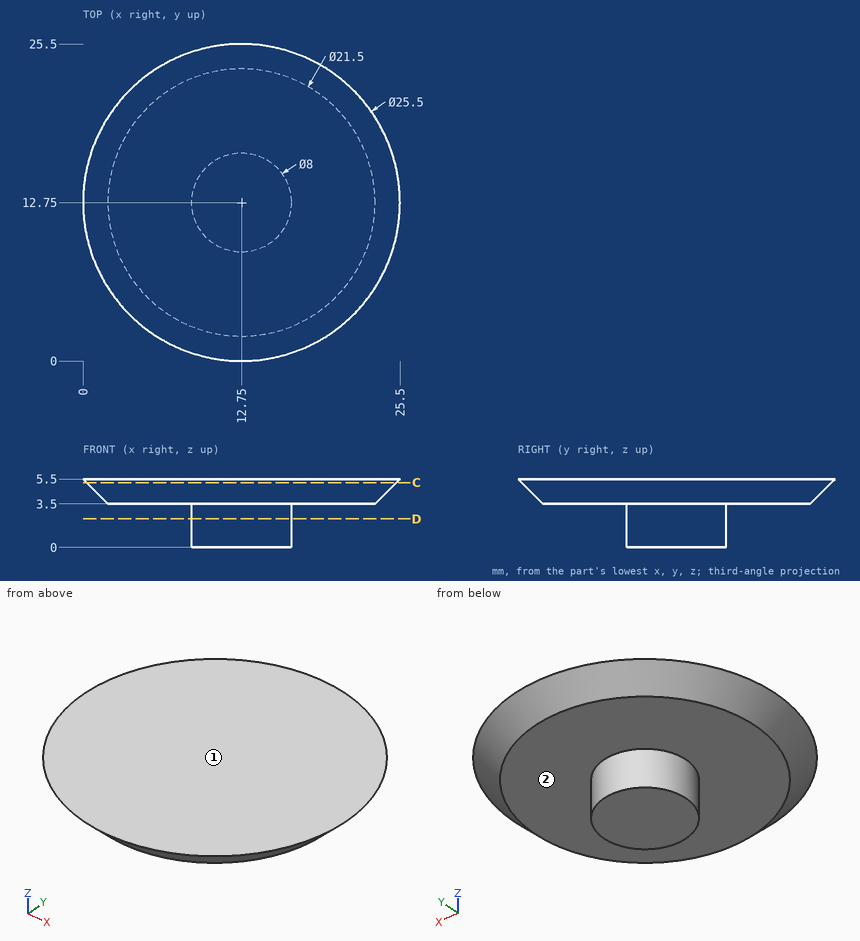
Input: dimensioned drawing with shaded views. Units: mm. Origin: part minimum x, y, z. A direction names the side the tool comes from. Give positions to 0.01 mm unless a question says otherwise; leave off trailing zeros. Loops run counter-clockwise (first coordinate to the right, second up) from the corner with the lowest first, then second, coordinate; pieces in that order, holes last. Notation, with made-up numbers: M -19,-5 L 26,-5 A30 ccw 26,30 Z; hole C 62,29 d10. An arc over 180 degrees is marked long. Put each result on its own line as item: value. Start each with the question number.
1) Contact query for flat-ended pins moving along their axis: pin 1 (4 mm diameter, centred on x = 20.5, y = 7.5, fed in from -Z); pin 2 (11 mm diameter, centred on x = 8, y = 13, fed in from -Z); pin 3 (1 mm diameter, centred on x = 17, z = 4.5, fed in from -Y). Output: stop coordinate, or through.
2) Cut plane C-C (z = 5.2). Output: boundary loops of the cut face in (x, y), then the cut area to 3 significant figures.
3) Cut plane D-D (z = 2.3). Output: boundary loops of the cut face in (x, y).
4) Ray query, line 1 along Z through (x, y) = (17.5, 14); line 2 along Y through (x, z) = (17.25, 4.4); line 3 along Y through (x, z) = (15.25, 0.4). Return the intervals inside material, ascending.
5) Access query for the marked faces 1 and 2. Directions: +Z, -Z, +X, -X, +Y, -Y. A direction counts if a zero-diameter tool reaches every point of the face in a straight line with its end or side. Return the directions, or none.
Verdict:
1. pin 1: z = 3.5
1. pin 2: z = 0
1. pin 3: y = 1.23
2. outline: C 12.75,12.75 d24.9
2. area: 487 mm2
3. outline: C 12.75,12.75 d8
4. line 1: 3.5 to 5.5
4. line 2: 2 to 23.5
4. line 3: 9.63 to 15.87
5. face 1: +Z, +X, -X, +Y, -Y
5. face 2: -Z
